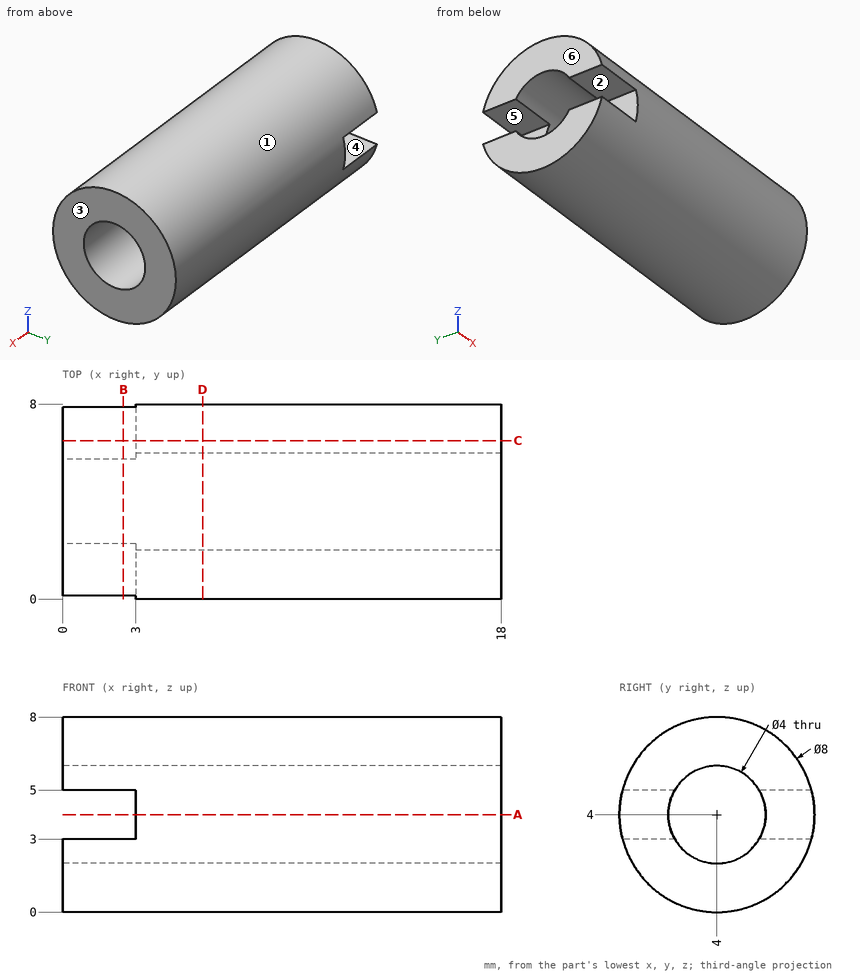
Source: three-view drawing plus pictorial views. Frame: mm from the lowest corner of the part. A direction names the side the tool comes from. Coordinates: 2 decimals unless noted, no trailing zeros. Order: outer loops, then holes, each group sorted by start corner. A loop starts at its lowest first (then second) coordinate and runs counter-clockwise, first axis right, second up. Notation, with made-up numbers: M 63,22.5 L 95,22.5 A13 ccw 95,45.5 Z; hole C 66.5,-6.75 d11. An arc over 180 degrees is marked long. Write each question's results on one line, items separated by ' | '. Start each with the question number.
1. Pin query (flat end, axial travel): pin 1 (0.6 mm diameter, centred on y = 6.5, z = 4, fed in from -X); pin 2 (4 mm diameter, centred on y = 5, z = 4.5, fed in from +X); pin 3 (3 mm diameter, centred on y = 4, z = 4, fed in from -X) (3 decimals); pin 4 (3 mm diameter, centred on x = 13.5, z = 2, fed in from +Y). Return the tip coordinate at first contact, or that it passes through.
2. Section D-D, the plane x = 5.75. Return the cut outline in (y, z).
3. Draft query along Z for the marked faces 1, 2, 3 and 4. Return one class per face: +Z half, -Z half, draft (parallel to the pull), parting line (faces both ways), or undercut.
4. Reachability of the marked faces 5 and 6 from +Z, -Z, +X, -X, +Y, -Y: full face, straight path, thin tool, end or side. Return the list, or none.
5. Section B-B, the plane x = 2.5. Return the cut outline in (y, z), then the cut area to 3 significant figures.
6. Section C-C, the plane y = 6.5. Return the cut outline in (x, z), then the cut area to 3 significant figures.
7. Material intervals for L1, parallel to Z at x = 12.5, y = 3; L2, parallel to Z at x = 4.5, y = 4, sorted ascending.
8. Section A-A, the plane z = 4. Return the cut outline in (x, y), then the cut area to 3 significant figures.
Solution:
1) pin 1: x = 3 | pin 2: x = 18 | pin 3: through | pin 4: y = 7.97
2) outline: C 4,4 d8; hole C 4,4 d4
3) face 1: parting line | face 2: undercut | face 3: draft | face 4: undercut
4) face 5: -X, +Y, -Y | face 6: +Z, -Z, -X, +Y, -Y
5) outline: M 0.13,3 A4 ccw 7.87,3 L 5.73,3 A2 cw 2.27,3 Z; M 0.13,5 L 2.27,5 A2 cw 5.73,5 L 7.87,5 A4 ccw Z | area: 29.5 mm²
6) outline: M 0,0.88 L 18,0.88 L 18,7.12 L 0,7.12 L 0,5 L 3,5 L 3,3 L 0,3 Z | area: 106 mm²
7) L1: 0.13 to 2.27, 5.73 to 7.87 | L2: 0 to 2, 6 to 8
8) outline: M 3,0 L 18,0 L 18,2 L 3,2 Z; M 3,6 L 18,6 L 18,8 L 3,8 Z | area: 60.0 mm²
